from build123d import *

# Parameters (mm, degrees)
BOSS_EXTRUDE1_DEPTH = 19.05
FILLET1_R           = 0.5
SKETCH3_R           = 2.75
CUT_EXTRUDE1_DEPTH  = 45.418274674
SKETCH4_R           = 2.75
CUT_EXTRUDE2_DEPTH  = 45.500933979


with BuildPart() as part:
    # Sketch1 → Boss-Extrude1 (new body)
    with BuildSketch(Plane.XY):
        Polygon((0, 0), (9.475, 0), (9.475, 3.175), (30.525, 3.175), (30.525, 0), (40, 0), (40, -1), (29.525, -1), (29.525, 2.175), (10.475, 2.175), (10.475, -1), (0, -1), align=None)
    extrude(amount=-BOSS_EXTRUDE1_DEPTH)

    # Fillet1
    fillet1_edges = [part.edges().sort_by_distance(p)[0] for p in [
        (9.475, 0, -9.525),
        (9.475, 3.175, -9.525),
        (30.525, 3.175, -9.525),
        (30.525, 0, -9.525),
        (29.525, -1, -9.525),
        (29.525, 2.175, -9.525),
        (10.475, 2.175, -9.525),
        (10.475, -1, -9.525),
    ]]
    fillet(fillet1_edges, radius=FILLET1_R)

    # Sketch3 → Cut-Extrude1 (cut, through all)
    with BuildSketch(Plane(origin=(0, 0, 0), x_dir=(1, 0, 0), z_dir=(0, 1, 0))):
        with Locations(Location((5, 9.525, 0), (0, 0, 270))):
            Circle(SKETCH3_R)
        with Locations(Location((35, 9.525, 0), (0, 0, 90))):
            Circle(SKETCH3_R)
    extrude(amount=-CUT_EXTRUDE1_DEPTH, mode=Mode.SUBTRACT)

    # Sketch4 → Cut-Extrude2 (cut, through all)
    with BuildSketch(Plane(origin=(0, 3.175, 0), x_dir=(1, 0, 0), z_dir=(0, 1, 0))):
        with Locations(Location((20, 9.525, 0), (0, 0, 270))):
            Circle(SKETCH4_R)
    extrude(amount=-CUT_EXTRUDE2_DEPTH, mode=Mode.SUBTRACT)


solid = part.part
The listing builds one solid part. Answer for the finished solid, in the listing's coordinates (mm). A direction names the side the tool comes from. Round coordinates to 2 decimals unless told otherwise and drop trailing zeros. Write each loop counter-clockwise with the first axis right and the second up, starting at its lowest first coordinate (ties: lowest second). Pieces come first, ordered by that corner, then holes. Notation, with made-up numbers: (7, 72) - (13, 72) arc R24 cw to (13, 105) - close; hole circle Ø2 at (89, -35). An arc over 180 degrees is marked (long way). Use a Markdown table: item, result. Add a question column.
1. The part is cut by section A-A (x = 35). Write down the section's boundary in (y, z) (3 decimals), and give its area (4 significant figures).
2. The part is cut by section D-D (x = 7). Write down the section's boundary in (y, z), and give its area (3 significant figures).
3. For a pull along Z with two mould halves and no side action, classify faces 5 (the face through (22.727, 2.682, -9.883)), 6 (the face through (9.475, 2, -9)), 7 (the face through (20.1, 2.5, 0)) as +Z half, -Z half, draft (parallel to the pull), parting line (faces both ways), or undercut.
4. The part is cut by section C-C (z = -7.5). Give the number of separate pieces and of enclosed holes in the cut face, and give its area (3 significant figures).
5. A tool of negligible diameter and unlimited length cuts with its end or side. For faces 1 (the face through (37, -1, -12)), 2 (the face through (30.525, 2, -9)), 3 (the face through (29.525, 1, -9)), 4 (the face through (2, 0, -12)), from which of +Z, -Z, +X, -X, +Y, -Y can it reach the whole face along a straight path? Write none if from no direction.
6. Consider line 1 (X direction, y = 1.45, z = -3.25) (3 decimals); line 2 (X direction, y = -0.55, z = -10.75); line 3 (Y direction, x = 11.5, z = -11.75) (3 decimals). Determine where each line is inside the solid, lowest interval first.
7. The part is cut by section B-B (z = -12.75). Write down the section's boundary in (x, y) (3 decimals).
8. Flat-ended cylindrical pins translate along their axes: P1, Ø0.7, axis at y = 1, z = -7, coming from the +X side (3 decimals); P2, Ø2.5, axis at x = 36.5, z = -14.5, coming from the +Y side; P3, Ø1, axis at x = 34.5, z = -12, coming from the -Y side; P4, Ø1.7, axis at y = 1.5, z = -5.5, coming from the -X side (3 decimals). Find the tip coordinate at first contact, or state that the pin passes through.
Reported:
| question | item | result |
|---|---|---|
| 1 | outline | (-1, -19.05) - (0, -19.05) - (0, -12.275) - (-1, -12.275) - close; (-1, -6.775) - (0, -6.775) - (0, 0) - (-1, 0) - close |
| 1 | area | 13.55 mm^2 |
| 2 | outline | (-1, -19.05) - (0, -19.05) - (0, -11.41) - (-1, -11.41) - close; (-1, -7.64) - (0, -7.64) - (0, 0) - (-1, 0) - close |
| 2 | area | 15.3 mm^2 |
| 3 | face 5 | undercut |
| 3 | face 6 | draft |
| 3 | face 7 | +Z half |
| 4 | separate pieces | 4 |
| 4 | enclosed holes | 0 |
| 4 | area | 35.2 mm^2 |
| 5 | face 1 | +Z, -Z, +X, -X, -Y |
| 5 | face 2 | +Z, -Z, +X, +Y |
| 5 | face 3 | +Z, -Z, -Y |
| 5 | face 4 | +Z, -Z, -X, +Y |
| 6 | line 1 | 9.475 to 10.475, 29.525 to 30.525 |
| 6 | line 2 | 0 to 2.54, 7.46 to 10.47, 29.53 to 32.54, 37.46 to 40 |
| 6 | line 3 | 2.175 to 3.175 |
| 7 | outline | (0, -1) - (9.975, -1) arc R0.5 ccw to (10.475, -0.5) - (10.475, 1.675) arc R0.5 cw to (10.975, 2.175) - (29.025, 2.175) arc R0.5 cw to (29.525, 1.675) - (29.525, -0.5) arc R0.5 ccw to (30.025, -1) - (40, -1) - (40, 0) - (31.025, 0) arc R0.5 cw to (30.525, 0.5) - (30.525, 2.675) arc R0.5 ccw to (30.025, 3.175) - (9.975, 3.175) arc R0.5 ccw to (9.475, 2.675) - (9.475, 0.5) arc R0.5 cw to (8.975, 0) - (0, 0) - close |
| 8 | P1 | x = 30.525 |
| 8 | P2 | y = 0 |
| 8 | P3 | y = -1 |
| 8 | P4 | x = 9.475 |
